Source: three-view drawing plus pictorial views. Frame: mm from the lowest corner of the part. A direction names the side the tool comes from. Give positions to 0.01 mm unless a question says otherwise; leave off trailing zeros. Write each loop counter-clockwise with the first axis right and the second up, starting at its lowest first coordinate (ties: lowest second). Pieces come first, ordered by that corner, then holes.
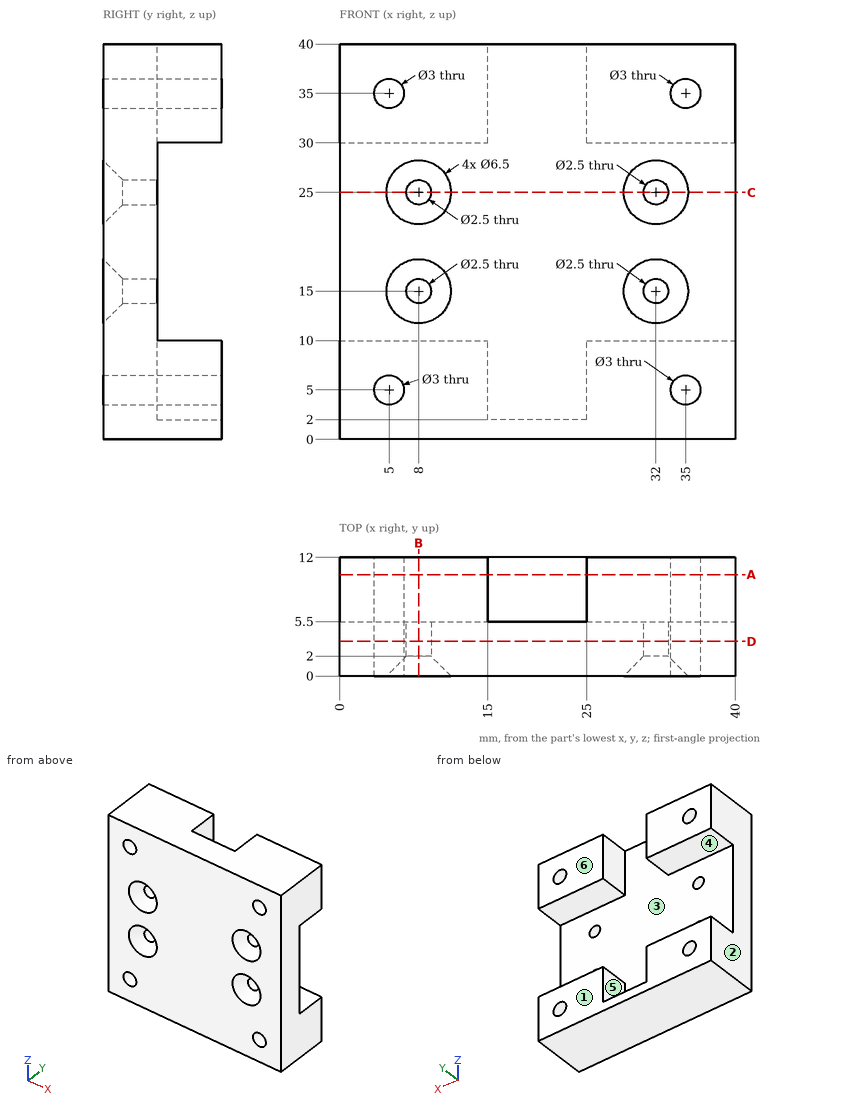
Q1. Section C-C on z = 25. Output: boundary loops of the cut face in (x, y), plus the area to 4 significant figures.
Filled sheet:
outline: (0, 0) - (4.75, 0) - (6.75, 2) - (6.75, 5.5) - (0, 5.5) - close; (9.25, 2) - (11.25, 0) - (28.75, 0) - (30.75, 2) - (30.75, 5.5) - (9.25, 5.5) - close; (33.25, 2) - (35.25, 0) - (40, 0) - (40, 5.5) - (33.25, 5.5) - close
area: 184.5 mm2
Q2. Pin query (flat end, axial travel): P1, Ø1, axis at x = 25.5, z = 11, coming from the +Y side; P2, Ø2.5, axis at x = 35, z = 35, coming from the +Y side (3 decimals). Return the tip coordinate at first contact, or that it passes through.
Filled sheet:
P1: stops at y = 5.5
P2: passes through
Q3. Section B-B on x = 8. Output: boundary loops of the cut face in (y, z).
Filled sheet:
outline: (0, 0) - (12, 0) - (12, 10) - (5.5, 10) - (5.5, 13.75) - (2, 13.75) - (0, 11.75) - close; (0, 18.25) - (2, 16.25) - (5.5, 16.25) - (5.5, 23.75) - (2, 23.75) - (0, 21.75) - close; (0, 28.25) - (2, 26.25) - (5.5, 26.25) - (5.5, 30) - (12, 30) - (12, 40) - (0, 40) - close
Q4. Ray query, line 1 along Z through (x, y) = (35, 4); line 2 along X through (y, z) = (2.9, 25); line 3 along X through (y, z) = (7.75, 35). Return the intervals inside material, ascending.
Filled sheet:
line 1: z = 0 to 3.5, 6.5 to 33.5, 36.5 to 40
line 2: x = 0 to 6.75, 9.25 to 30.75, 33.25 to 40
line 3: x = 0 to 3.5, 6.5 to 15, 25 to 33.5, 36.5 to 40
Q5. Section D-D on y = 3.5. Count the separate pieces of the cut face and the enclosed holes in it, plus the area to 3 significant figures.
Filled sheet:
separate pieces: 1
enclosed holes: 8
area: 1,550 mm2
Q6. Pull-direction query (X, two-part tool) for the marked faces 1, 2 and 3; classes: released by +X, released by -X, zero draft, split by the parting line, or undercut.
Filled sheet:
face 1: zero draft
face 2: released by -X
face 3: undercut
Q7. Section A-A on y = 10.25. Output: boundary loops of the cut face in (x, z).
Filled sheet:
outline: (0, 0) - (40, 0) - (40, 10) - (25, 10) - (25, 2) - (15, 2) - (15, 10) - (0, 10) - close; (0, 30) - (15, 30) - (15, 40) - (0, 40) - close; (25, 30) - (40, 30) - (40, 40) - (25, 40) - close; hole circle Ø3 at (5, 5); hole circle Ø3 at (5, 35); hole circle Ø3 at (35, 5); hole circle Ø3 at (35, 35)
Q8. Access query for the marked faces 4, 5 and 6. Directions: +Z, -Z, +X, -X, +Y, -Y. A direction counts if a zero-diameter tool reaches every point of the face in a straight line with its end or side. Return the directions, or none.
Filled sheet:
face 4: +X, -X, +Y
face 5: +Z, +Y
face 6: +Z, -Z, +X, -X, +Y
